from build123d import *

# Parameters (mm, degrees)
SKETCH1_R           = 25
BOSS_EXTRUDE1_DEPTH = 39
SKETCH2_R           = 23.5
BOSS_EXTRUDE2_DEPTH = 50
SKETCH3_R           = 5
BOSS_EXTRUDE3_DEPTH = 20
SKETCH4_W           = 4.717886869
SKETCH4_H           = 0.61518364
SKETCH4_H_2         = 1.339282812
BOSS_EXTRUDE4_DEPTH = 5


with BuildPart() as part:
    # Sketch1 → Boss-Extrude1 (new body)
    with BuildSketch(Plane.XY):
        Circle(SKETCH1_R)
    extrude(amount=BOSS_EXTRUDE1_DEPTH)

    # Sketch2 → Boss-Extrude2 (add)
    with BuildSketch(Plane.XY.offset(39)):
        Circle(SKETCH2_R)
    extrude(amount=BOSS_EXTRUDE2_DEPTH)

    # Sketch3 → Boss-Extrude3 (add)
    with BuildSketch(Plane.XY.offset(89)):
        Circle(SKETCH3_R)
    extrude(amount=BOSS_EXTRUDE3_DEPTH)

    # Sketch4 → Boss-Extrude4 (add)
    with BuildSketch(Plane(origin=(0, 0, 0), x_dir=(0, 0, -1), z_dir=(1, 0, 0))):
        with Locations((2.358943434, 24.69240818)):
            Rectangle(SKETCH4_W, SKETCH4_H)
        with Locations((2.358943434, -24.848693341)):
            Rectangle(SKETCH4_W, SKETCH4_H_2)
    extrude(amount=BOSS_EXTRUDE4_DEPTH)


solid = part.part
Geometry check sheet. Reference: the model listing, model coordinates, mm. A direction names the side the tool comes from. Round coordinates to 2 decimals unless told otherwise and drop trailing zeros. Write each loop counter-clockwise with the first axis right and the second up, starting at its lowest first coordinate (ties: lowest second). Pieces come first, ordered by that corner, then holes. Notation, with made-up numbers: (-6.5, 56.25) - (50.5, 56.25) arc R16 ccw to (50.5, 73.25) - close; hole circle Ø11 at (48.25, 13). An arc over 180 degrees is marked (long way). One line per item, written item: value.
1. Cross-section at B-B on z = 63. Record the boundary of the cut face in (x, y), and give its area (3 significant figures).
The answers:
outline: circle Ø47 at (0, 0)
area: 1,730 mm^2
2. Cross-section at C-C on x = 7. Record the boundary of the cut face in (y, z).
The answers:
outline: (-24, 0) - (24, 0) - (24, 39) - (22.43, 39) - (22.43, 89) - (-22.43, 89) - (-22.43, 39) - (-24, 39) - close
3. Cross-section at D-D on y = -22. Record the boundary of the cut face in (x, z).
The answers:
outline: (-11.87, 0) - (11.87, 0) - (11.87, 39) - (8.26, 39) - (8.26, 89) - (-8.26, 89) - (-8.26, 39) - (-11.87, 39) - close
4. Depth check by flat-ended pin: pin 1 Ø3 at (x, z) = (2, 44.5) entering from +Y; pin 2 Ø1.5 at (x, y) = (-14, 7.5) entering from +Z; pin 3 Ø1.1 at (y, z) = (-25, -1.5) entering from +X; pin 4 Ø23.5 at (x, y) = (8, -2.5) entering from +Z. Enter the tip coordinate at first touch or a pass-through.
The answers:
pin 1: stops at y = 23.49
pin 2: stops at z = 89
pin 3: stops at x = 5
pin 4: stops at z = 109
5. Mould release check, pull along Y, two halves, no side actions. Record for faces 4 (the face through (-17, -17, 39)), 5 (the face through (2, 24.385, -2)), 6 (the face through (23.846, 7.509, 19.227)): released by +Y, released by -Y, zero draft, split by the parting line, or undercut.
The answers:
face 4: zero draft
face 5: undercut
face 6: split by the parting line
6. Set-up check for faces 1 (the face through (2, -24.179, -2)), 2 (the face through (2, -25.518, -2)), 3 (the face through (22.4, 7.1, 63.6)): record each of +Z, -Z, +X, -X, +Y, -Y from which the full face is reachable in a straight line by a thin tool's end or side.
The answers:
face 1: -Z, +X, -X
face 2: +Z, -Z, +X, -X, -Y
face 3: +Z
7. Cross-section at A-A on y = 0. Record the boundary of the cut face in (x, z), and give its area (3 significant figures).
The answers:
outline: (-25, 0) - (25, 0) - (25, 39) - (23.5, 39) - (23.5, 89) - (5, 89) - (5, 109) - (-5, 109) - (-5, 89) - (-23.5, 89) - (-23.5, 39) - (-25, 39) - close
area: 4,500 mm^2
8. Scan lines: L1, parallel to Y at x = -0.5, z = 43; L2, parallel to Z at x = -1, y = 17.5; L3, parallel to Y at x = -15, z = 86. Record each from-to range of solid material in increasing order.
The answers:
L1: y = -23.49 to 23.49
L2: z = 0 to 89
L3: y = -18.09 to 18.09
